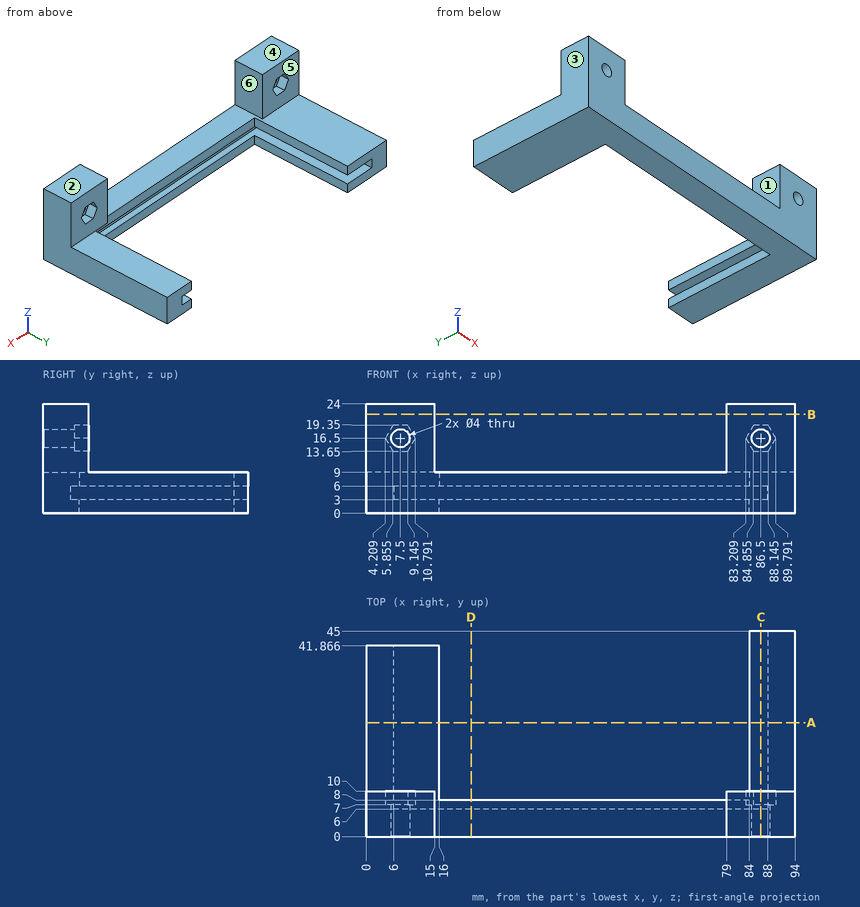
Geometry check sheet. Reference: drawing and pictorial views, mm from the part's lowest x, y, z. A direction names the side the tool comes from. Round coordinates to 2 decimals unless told otherwise and drop trailing zeros. Write each loop counter-clockwise with the first axis right and the second up, starting at its lowest first coordinate (ties: lowest second). Pieces come first, ordered by that corner, then holes.
1. Section check D-D on x = 23. Enter the section's corners in (y, z).
2. Draft check along X on the marked faces 1, 2 and 3. Enter one of: +X half, -X half, draft (parallel to the pull), parting line (faces both ways), or undercut.
3. Scan lines: L1, parallel to X at y = 2, z = 16.5; L2, parallel to X at y = 39, z = 2.75; L3, parallel to Z at x = 86.5, y = 1.75. Record each from-to range of solid material in increasing order.
4. Section check A-A on y = 25. Enter the section's corners in (x, z).
5. Section check B-B on z = 21.75. Enter the section's corners in (x, y), plus the area to 3 significant figures.
6. Gauge pin test, flat ends, axial feed: P1, Ø1, axis at x = 61, z = 4, coming from the +Y side; P2, Ø4.5, axis at x = 6, z = 15.5, coming from the +Y side; P3, Ø5, axis at x = 57, y = 9.5, coming from the +Z side; P4, Ø1, axis at x = 33, z = 11, coming from the +Y side. Record the tip position at first contact, or that the pin passes through.
7. Section check C-C on x = 86.5. Enter the section's corners in (y, z).
8. Access from +Z, -Z, +X, -X, +Y, -Y to the whole of each face (thin tool, end or side, straight path). Record for the marked faces 4, 5 and 6.
Answer:
1. outline: (0, 0) - (8, 0) - (8, 3) - (6, 3) - (6, 6) - (8, 6) - (8, 9) - (0, 9) - close
2. face 1: undercut
2. face 2: draft
2. face 3: -X half
3. L1: x = 0 to 5.5, 9.5 to 15, 79 to 84.5, 88.5 to 94
3. L2: x = 0 to 16, 84 to 94
3. L3: z = 0 to 14.5, 18.5 to 24
4. outline: (0, 0) - (16, 0) - (16, 3) - (6, 3) - (6, 6) - (16, 6) - (16, 9) - (0, 9) - close; (84, 0) - (94, 0) - (94, 9) - (84, 9) - (84, 6) - (88, 6) - (88, 3) - (84, 3) - close
5. outline: (0, 0) - (15, 0) - (15, 10) - (0, 10) - close; (79, 0) - (94, 0) - (94, 10) - (79, 10) - close
5. area: 300 mm2
6. P1: stops at y = 6
6. P2: stops at y = 10
6. P3: stops at z = 9
6. P4: passes through
7. outline: (0, 0) - (45, 0) - (45, 3) - (6, 3) - (6, 6) - (45, 6) - (45, 9) - (10, 9) - (10, 13.65) - (7, 13.65) - (7, 14.5) - (0, 14.5) - close; (0, 18.5) - (7, 18.5) - (7, 19.35) - (10, 19.35) - (10, 24) - (0, 24) - close
8. face 4: +Z, +X, -X, +Y, -Y
8. face 5: +Z, +X, -X, +Y
8. face 6: +Z, +Y, -Y
